Here's how the part is built. I have some questions about the finished solid (model axes, mm). A direction names the side the tool comes from. Round coordinates to 2 decimals unless told otherwise and drop trailing zeros. Order: outer loops, then holes, each group sorted by start corner. A loop starts at its lowest first (then second) coordinate and runs counter-clockwise, first axis right, second up. Notation, with made-up numbers: (17, -4) -> (43, -4) arc R34 cw to (43, 29) -> close; hole circle Ø3 at (79, -10.75). An arc over 180 degrees is marked (long way). One line per item, written item: value.
```python
from build123d import *

# Parameters (mm, degrees)
SKETCH1_W           = 47
SKETCH1_H           = 52
BOSS_EXTRUDE1_DEPTH = 50
SKETCH8_W           = 25
SKETCH8_H           = 16
CUT_EXTRUDE1_DEPTH  = 10
CUT_EXTRUDE2_START  = -2
CUT_EXTRUDE2_DEPTH  = 3.5
CUT_EXTRUDE3_DEPTH  = 3.5
CHAMFER1_SIZE       = 1
SKETCH6_W           = 53
SKETCH6_H           = 58
SKETCH6_W_2         = 47
SKETCH6_H_2         = 52
BOSS_EXTRUDE3_DEPTH = 74
CHAMFER2_SIZE       = 1


with BuildPart() as part:
    # Sketch1 → Boss-Extrude1 (new body)
    with BuildSketch(Plane.XY):
        Polygon((17.540775456, -97.544656267), (17.540775456, -113.544656267), (9.540775456, -113.544656267), (9.540775456, -35.544656267), (69.540775456, -35.544656267), (69.540775456, -97.544656267), align=None)
        with Locations((41.040775456, -66.544656267)):
            Rectangle(SKETCH1_W, SKETCH1_H, mode=Mode.SUBTRACT)
    extrude(amount=BOSS_EXTRUDE1_DEPTH)

    # Sketch8 → Cut-Extrude1 (cut)
    with BuildSketch(Plane(origin=(17.540775456, 0, 0), x_dir=(0, 0, -1), z_dir=(1, 0, 0))):
        with Locations((-37.5, -105.544656267)):
            Rectangle(SKETCH8_W, SKETCH8_H)
    extrude(amount=-CUT_EXTRUDE1_DEPTH, mode=Mode.SUBTRACT)

    # Sketch9 → Cut-Extrude2 (cut)
    with BuildSketch(Plane.ZY.offset(-9.540775456).offset(CUT_EXTRUDE2_START)):
        with BuildLine():
            Line((35, -49.794656267), (28, -49.794656267))
            ThreePointArc((28, -49.794656267), (24.25, -46.044656267), (28, -42.294656267))
            Line((28, -42.294656267), (35, -42.294656267))
            ThreePointArc((35, -42.294656267), (38.75, -46.044656267), (35, -49.794656267))
        make_face()
        with BuildLine():
            Line((15, -106.794656267), (8, -106.794656267))
            ThreePointArc((8, -106.794656267), (4.25, -103.044656267), (8, -99.294656267))
            Line((8, -99.294656267), (15, -99.294656267))
            ThreePointArc((15, -99.294656267), (18.75, -103.044656267), (15, -106.794656267))
        make_face()
    extrude(amount=-CUT_EXTRUDE2_DEPTH, mode=Mode.SUBTRACT)

    # Sketch10 → Cut-Extrude3 (cut)
    with BuildSketch(Plane.ZY.offset(-9.540775456)):
        with BuildLine():
            Line((35, -48.094656267), (32.478839135, -48.094656267))
            ThreePointArc((32.478839135, -48.094656267), (31.41425784, -48.289898404), (30.488243964, -48.850211822))
            ThreePointArc((30.488243964, -48.850211822), (24.25, -46.044656267), (30.488243964, -43.239100711))
            ThreePointArc((30.488243964, -43.239100711), (31.41425784, -43.799414129), (32.478839135, -43.994656267))
            Line((32.478839135, -43.994656267), (35, -43.994656267))
            ThreePointArc((35, -43.994656267), (37.05, -46.044656267), (35, -48.094656267))
        make_face()
        with BuildLine():
            Line((12.478839135, -100.994656267), (15, -100.994656267))
            ThreePointArc((15, -100.994656267), (17.05, -103.044656267), (15, -105.094656267))
            Line((15, -105.094656267), (12.478839135, -105.094656267))
            ThreePointArc((12.478839135, -105.094656267), (11.41425784, -105.289898404), (10.488243964, -105.850211822))
            ThreePointArc((10.488243964, -105.850211822), (4.25, -103.044656267), (10.488243964, -100.239100711))
            ThreePointArc((10.488243964, -100.239100711), (11.41425784, -100.799414129), (12.478839135, -100.994656267))
        make_face()
    extrude(amount=-CUT_EXTRUDE3_DEPTH, mode=Mode.SUBTRACT)

    # Chamfer1
    chamfer1_edges = [part.edges().sort_by_distance(p)[0] for p in [
        (69.540775456, -35.544656267, 25),
        (69.540775456, -97.544656267, 25),
        (39.540775456, -35.544656267, 50),
        (17.540775456, -66.544656267, 50),
        (41.040775456, -92.544656267, 50),
        (64.540775456, -66.544656267, 50),
        (41.040775456, -40.544656267, 50),
        (17.540775456, -97.544656267, 12.5),
        (17.540775456, -113.544656267, 12.5),
        (13.540775456, -97.544656267, 25),
        (17.540775456, -105.544656267, 25),
        (39.540775456, -97.544656267, 50),
        (69.540775456, -66.544656267, 50),
    ]]
    chamfer(chamfer1_edges, length=CHAMFER1_SIZE)

    # Sketch6 → Boss-Extrude3 (add)
    with BuildSketch(Plane(origin=(0, 0, 0), x_dir=(-1, 0, 0), z_dir=(0, 0, -1))):
        with Locations((-41.040775456, -66.544656267)):
            Rectangle(SKETCH6_W, SKETCH6_H)
        with Locations((-41.040775456, -66.544656267)):
            Rectangle(SKETCH6_W_2, SKETCH6_H_2, mode=Mode.SUBTRACT)
    extrude(amount=BOSS_EXTRUDE3_DEPTH)

    # Chamfer2
    chamfer2_edges = [part.edges().sort_by_distance(p)[0] for p in [
        (67.540775456, -66.544656267, 0),
        (41.040775456, -95.544656267, 0),
        (14.540775456, -66.544656267, 0),
        (41.040775456, -37.544656267, 0),
    ]]
    chamfer(chamfer2_edges, length=CHAMFER2_SIZE)


solid = part.part
```
Q1. For P1, Ø12, axis at x = 39.5, z = 31, coming from the -Y side; P2, Ø12, axis at x = 50, y = -89.5, coming from the +Z side; P3, Ø3.5, axis at x = 13, y = -106, coming from the +Z side; P4, Ø3, axis at x = 20, y = -75, coming from the +Z side, each with a flat end and sliding along its axis, tell me the tip position at first contact or that it passes through.
Answers:
P1: y = -97.54
P2: z = 50
P3: z = 25
P4: through
Q2. I need wall thicknesses on line 1 along Y through (x, z) = (13, 8); line 2 along Y through (x, z) = (19, -3.5); line 3 along X through (y, z) = (-54, -47). Which ranges of each line are inside material? Lowest first, please.
Answers:
line 1: -113.54 to -106.79, -99.29 to -35.54
line 2: -95.54 to -92.54, -40.54 to -37.54
line 3: 14.54 to 17.54, 64.54 to 67.54
Q3. I want a section at C-C on x = 30. Write out the boundary of the cut face in (y, z).
Answers:
outline: (-97.54, 0) -> (-96.54, 0) -> (-95.54, -1) -> (-95.54, -74) -> (-92.54, -74) -> (-92.54, 49) -> (-93.54, 50) -> (-96.54, 50) -> (-97.54, 49) -> close; (-40.54, -74) -> (-37.54, -74) -> (-37.54, -1) -> (-36.54, 0) -> (-35.54, 0) -> (-35.54, 49) -> (-36.54, 50) -> (-39.54, 50) -> (-40.54, 49) -> close
Q4. Which directions (+Z, -Z, +X, -X, +Y, -Y) give clear straight access to the entire face, cutting with the end or side of a thin tool? Please do faces 5 (the face through (41, -95.545, -37)), 6 (the face through (67.541, -67, -37)), 7 (the face through (13, -106, 25)), 8 (the face through (13, -42.295, 31)), 9 (the face through (41, -40.545, -12)).
Answers:
face 5: -Z, +X, -X, -Y
face 6: -Z, +X, +Y, -Y
face 7: +Z, +X, -X, -Y
face 8: none
face 9: +Z, -Z
Q5. If we mould it in two halves opening along Z, with no side actions, what happens to faces 1 (the face through (65, -66, -74)), 2 (the face through (13.27, -45.96, 38.75)), 3 (the face through (14.541, -67, -37)), 4 (the face through (11.541, -48.5, 34.6))? For each: pulls with the +Z half, pulls with the -Z half, needs draft (parallel to the pull), parting line crosses it, or undercut.
Answers:
face 1: pulls with the -Z half
face 2: undercut
face 3: needs draft
face 4: undercut
Q6. I want a section at B-B on z = -25.5. Write out the boundary of the cut face in (x, y).
Answers:
outline: (14.54, -95.54) -> (67.54, -95.54) -> (67.54, -37.54) -> (14.54, -37.54) -> close; hole (17.54, -92.54) -> (64.54, -92.54) -> (64.54, -40.54) -> (17.54, -40.54) -> close
Q7. I want a section at A-A on y = -85. Write out the boundary of the cut face in (x, z), then the cut area to 3 significant figures.
Answers:
outline: (9.54, 0) -> (13.54, 0) -> (14.54, -1) -> (14.54, -74) -> (17.54, -74) -> (17.54, 49) -> (16.54, 50) -> (9.54, 50) -> close; (64.54, -74) -> (67.54, -74) -> (67.54, -1) -> (68.54, 0) -> (69.54, 0) -> (69.54, 49) -> (68.54, 50) -> (65.54, 50) -> (64.54, 49) -> close
area: 1,090 mm2
